Input: part model. Units: mm. Frame: model coordinates. A direction names the side the tool comes from. Give positions to 0.01 mm unless a question says otherwise; leave off trailing zeros. Order: outer loops, then holes, each group sorted by start corner. A loop starts at its lowest first (then second) coordinate and runs counter-clockwise, first axis right, second up. Notation, with made-up numbers: (28.5, 10.25) - (54.5, 10.25) arc R26 cw to (54.5, 29.25) - close; hole circle Ø1 at (77.5, 15). An arc over 180 degrees is marked (long way). Answer in a Markdown table with one row per item. Add a question column.
1. Section query C-C on z = 47.5. Return loops of the section in (x, y).
2. Access query for faces 4 (the face through (13, 0, 538)), 5 (the face through (12.88, -138.94, 22.9)), 6 (the face through (12.878, -10.837, -20.303)). Directions: +Z, -Z, +X, -X, +Y, -Y. A direction counts if a zero-diameter tool reaches every point of the face in a straight line with its end or side. Return the directions, or none.
3. Contact query for flat-ended pins moving along their axis: pin 1 (8 mm diameter, centred on x = 3.5, z = 295, fed in from -Y); pin 2 (12 mm diameter, centred on x = 19, y = -36, fed in from +Z); pin 3 (12 mm diameter, centred on x = 19.5, y = -265.5, fed in from -Z). Output: stop coordinate, or through.
4. Ray query, line 1 (Y direction, x = 16.5, z = 226.5); line 2 (Z direction, x = 16, y = -155.5); line 3 (Z direction, x = 15, y = -157.5). Return the intervals inside material, ascending. Write a range as [from, to].
5. Section query A-A on y = -156. Return loops of the section in (x, z).
6. Mould query, pull axis Y, two halves, no side actions, for faces 1 (the face through (12.878, -10.424, -19.726)), 2 (the face through (13, 0.254, 538)), 3 (the face through (12.88, -142.04, 23.94)). Classes: released by +Y, released by -Y, zero draft, split by the parting line, or undercut.
7. Section query B-B on x = 8. Return loops of the section in (y, z).
```python
from build123d import *

# Parameters (mm, degrees)
SKETCH1_W           = 25.4
SKETCH1_H           = 0.254
BOSS_EXTRUDE1_DEPTH = 1091.946
BOSS_EXTRUDE4_DEPTH = 25.4


with BuildPart() as part:
    # Sketch1 → Boss-Extrude1 (new body)
    with BuildSketch(Plane.XY):
        with Locations((12.7, 0.127)):
            Rectangle(SKETCH1_W, SKETCH1_H)
    extrude(amount=BOSS_EXTRUDE1_DEPTH)

    # Sketch2 → Boss-Extrude4 (add)
    with BuildSketch(Plane(origin=(25.4, 0, 0), x_dir=(0, 0, -1), z_dir=(1, 0, 0))):
        with BuildLine():
            Line((21.978237679, -33.20447493), (-69.053498166, -247.6786673))
            ThreePointArc((-69.053498166, -247.6786673), (-235.384405248, -190.597617752), (-62.661653687, -223.628935639))
            Line((-62.661653687, -223.628935639), (-62.415163254, -223.707110938))
            ThreePointArc((-62.415163254, -223.707110938), (-235.623641363, -190.508902989), (-68.819687127, -247.777906395))
            Line((-68.819687127, -247.777906395), (22.212048718, -33.303714025))
            ThreePointArc((22.212048718, -33.303714025), (20.121476579, -10.557476047), (0, 0.254))
            Line((0, 0.254), (0, 0))
            ThreePointArc((0, 0), (19.909671562, -10.697671036), (21.978237679, -33.20447493))
        make_face()
    extrude(amount=-BOSS_EXTRUDE4_DEPTH)


solid = part.part
```
Answer:
| question | item | result |
|---|---|---|
| 1 | outline | (0, -197.55) - (25.4, -197.55) - (25.4, -196.9) - (0, -196.9) - close; (0, 0) - (25.4, 0) - (25.4, 0.25) - (0, 0.25) - close |
| 2 | face 4 | +Z, +X, -X |
| 2 | face 5 | +X, -X |
| 2 | face 6 | -Z, +X, -X |
| 3 | pin 1 | stops at y = 0 |
| 3 | pin 2 | stops at z = -18.25 |
| 3 | pin 3 | stops at z = 74.86 |
| 4 | line 1 | y = [-257.87, -257.37], [-169.11, -168.6], [0, 0.25] |
| 4 | line 2 | z = [29.65, 29.93], [83.25, 83.59], [216.8, 217.13] |
| 4 | line 3 | z = [30.5, 30.78], [81.58, 81.91], [218.48, 218.81] |
| 5 | outline | (0, 29.87) - (25.4, 29.87) - (25.4, 30.14) - (0, 30.14) - close; (0, 82.83) - (25.4, 82.83) - (25.4, 83.16) - (0, 83.16) - close; (0, 217.23) - (25.4, 217.23) - (25.4, 217.56) - (0, 217.56) - close |
| 6 | face 1 | undercut |
| 6 | face 2 | released by +Y |
| 6 | face 3 | released by -Y |
| 7 | outline | (-247.78, 68.82) - (-33.3, -22.21) arc R24.13 ccw to (0.25, 0) - (0.25, 1091.95) - (0, 1091.95) - (0, 0) arc R23.88 cw to (-33.2, -21.98) - (-247.68, 69.05) arc R88.15 cw (long way) to (-223.63, 62.66) - (-223.71, 62.42) arc R88.4 ccw (long way) to start |
